Geometry: final body of the model. Coordinates: model frame, mm. Face numbers are marked on the shaded views. A direction names the side the tool comes from. Coordinates: 2 decimals unless noted, no trailing zeros. Loops run counter-clockwise (first coordinate to the right, second up) from the corner with the lowest first, then second, coordinate; pieces in that order, holes last. Notation, with made-up numbers: (82.25, 43) -> (128.25, 43) arc R8 cw to (128.25, 47) -> close; hole circle Ø5 at (-38, 89.25). An arc over 180 degrees is marked (long way). One line per item, written item: value. Start each with the question number.
Item 1: Section query C-C on y = 22. Return loops of the section in (x, z) (3 decimals), then the cut area to 3 significant figures.
Item 2: Ray query, probe 1 along Y at (x, z) = (-57, -12); probe 2 along X at (y, z) = (17.5, 1.5); probe 3 along X at (y, z) = (28, 6.5). Return the intervals inside material, ascending. Write a range as from..to.
Item 3: Section query B-B on z = 0. Return loops of the section in (x, y) (3 decimals).
Item 4: Section query A-A on x = 0. Return loops of the section in (y, z) (3 decimals), then the cut area to 3 significant figures.
Item 5: Contact query for flat-ended pins moving along their axis: pin 1 Ø4 at (x, z) = (-51.5, -51) entering from -Y; pin 2 Ø12 at (x, z) = (55, 38.5) entering from +Y; pin 3 Ø12 at (x, y) = (3.5, 26) entering from -Z (3 decimals); pin 4 Ø12 at (y, z) = (8, -8.5) entering from +X. Output: stop coordinate, or through.
Item 6: Set-up query: the marked faces 1 and 2. Return all of +Z, -Z, +X, -X, +Y, -Y with unobstructed straight access to the full face (end or side cutting, diameter ignored); none if empty.
from build123d import *

# Parameters (mm, degrees)
SKETCH1_R           = 85.725
BOSS_EXTRUDE1_DEPTH = 6.35
SKETCH2_R           = 13.335
BOSS_EXTRUDE2_DEPTH = 35.56
FILLET1_R           = 2.54
FILLET2_R           = 2.54


with BuildPart() as part:
    # Sketch1 → Boss-Extrude1 (new body)
    with BuildSketch(Plane(origin=(0, 0, 0), x_dir=(1, 0, 0), z_dir=(0, 1, 0))):
        Circle(SKETCH1_R)
    extrude(amount=BOSS_EXTRUDE1_DEPTH)

    # Sketch2 → Boss-Extrude2 (add)
    with BuildSketch(Plane(origin=(0, 6.35, 0), x_dir=(1, 0, 0), z_dir=(0, 1, 0))):
        Circle(SKETCH2_R)
    extrude(amount=BOSS_EXTRUDE2_DEPTH)

    # Fillet1
    fillet1_edges = [part.edges().sort_by_distance(p)[0] for p in [
        (-13.335, 41.91, 0),
    ]]
    fillet(fillet1_edges, radius=FILLET1_R)

    # Fillet2
    fillet2_edges = [part.edges().sort_by_distance(p)[0] for p in [
        (-85.725, 6.35, 0),
    ]]
    fillet(fillet2_edges, radius=FILLET2_R)


solid = part.part
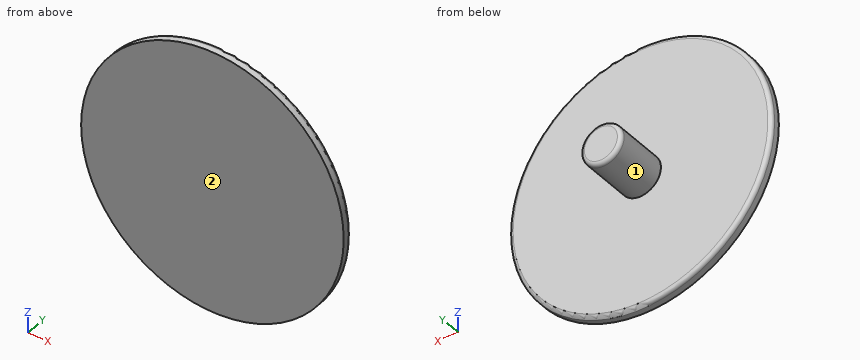
Reply:
1. outline: circle Ø26.67 at (0, 0)
1. area: 559 mm²
2. probe 1: y = 0..6.35
2. probe 2: x = -13.25..13.25
2. probe 3: x = -11.64..11.64
3. outline: (-85.725, 0) -> (85.725, 0) -> (85.725, 3.81) arc R2.54 ccw to (83.185, 6.35) -> (13.335, 6.35) -> (13.335, 39.37) arc R2.54 ccw to (10.795, 41.91) -> (-10.795, 41.91) arc R2.54 ccw to (-13.335, 39.37) -> (-13.335, 6.35) -> (-83.185, 6.35) arc R2.54 ccw to (-85.725, 3.81) -> close
4. outline: (0, -85.725) -> (3.81, -85.725) arc R2.54 ccw to (6.35, -83.185) -> (6.35, -13.335) -> (39.37, -13.335) arc R2.54 ccw to (41.91, -10.795) -> (41.91, 10.795) arc R2.54 ccw to (39.37, 13.335) -> (6.35, 13.335) -> (6.35, 83.185) arc R2.54 ccw to (3.81, 85.725) -> (0, 85.725) -> close
4. area: 2,030 mm²
5. pin 1: stops at y = 0
5. pin 2: stops at y = 6.35
5. pin 3: stops at z = -13.335
5. pin 4: stops at x = 85.62
6. face 1: +Y
6. face 2: +Z, -Z, +X, -X, -Y
